from build123d import *

# Parameters (mm, degrees)
F0_W      = 50.8
F0_H      = 30.48
F1_DEPTH  = 25.4
F2_DEPTH  = 55.626
F3_DEPTH  = 32.766
F6_DEPTH  = 25.4
F7_DEPTH  = 25.4
F9_DEPTH  = 25.4
F10_DEPTH = 7.62


with BuildPart() as f1:
    # F0 (on Front) → F1 (new body)
    with BuildSketch(Plane.XZ):
        with Locations((-32.1067409651, 15.24)):
            Rectangle(F0_W, F0_H)
    extrude(amount=F1_DEPTH)

    # F2 (add): a face of the model
    f2_faces = [f1.faces().sort_by_distance(p)[0] for p in [
        (-32.1067409651, 0, 15.24),
    ]]
    extrude(f2_faces, amount=F2_DEPTH)

    # F3 (add): a face of the model
    f3_faces = [f1.faces().sort_by_distance(p)[0] for p in [
        (-6.7067409651, 15.113, 15.24),
    ]]
    extrude(f3_faces, amount=F3_DEPTH)

    # F4 (on face) → F6 (cut)
    with BuildSketch(Plane.XY.offset(30.48)):
        Polygon((-11.3192433491, -25.4), (17.2114539891, 55.626), (-57.5067409651, 55.626), (-57.5067409651, -25.4), align=None)
    extrude(amount=-F6_DEPTH, mode=Mode.SUBTRACT)

    # F5 (on face) → F7 (cut)
    with BuildSketch(Plane.XY.offset(30.48)):
        Polygon((-57.5067409651, -25.4), (-11.3192433491, -25.4), (17.2114539891, 55.626), (-43.2823600247, 55.626), (-57.5067409651, 55.626), align=None)
    extrude(amount=-F7_DEPTH, mode=Mode.SUBTRACT)

    # F8 (on face) → F9 (join)
    with BuildSketch(Plane.XY.offset(5.08)):
        Polygon((-57.5067409651, 20.3126166016), (-36.7487818003, 55.626), (-57.5067409651, 55.626), align=None)
    extrude(amount=F9_DEPTH)

    # F10 (add): a face of the model
    f10_faces = [f1.faces().sort_by_distance(p)[0] for p in [
        (-24.788870281, 16.2328343869, 5.08),
    ]]
    extrude(f10_faces, amount=F10_DEPTH)


solid = f1.part
Could you check a few things on this model? Use its own coordinates, in mm. A direction names the side the tool comes from. Give positions to 0.01 mm unless a question says otherwise; leave off trailing zeros. Order: outer loops, then holes, each group sorted by start corner. A loop starts at its lowest first (then second) coordinate and runs counter-clockwise, first axis right, second up. Notation, with made-up numbers: M -10.75,15 L 2.25,15 A14 cw 2.25,22 Z; hole C -32,61.5 d10. An arc over 180 degrees is marked long. One line per question, with ' | ' between items.
1. I want a section at C-C (x = -7). List the corners of the cut face in (y, z) for me.
Results:
outline: M -25.4,0 L 55.63,0 L 55.63,12.7 L -13.13,12.7 L -13.13,30.48 L -25.4,30.48 Z
2. I want a section at B-B (y = 34.5). List the corners of the cut face in (x, z) for me, and give its area (3 significant figures).
Results:
outline: M -57.51,0 L 26.06,0 L 26.06,30.48 L 9.77,30.48 L 9.77,12.7 L -49.17,12.7 L -49.17,30.48 L -57.51,30.48 Z | area: 1,500 mm²
3. If I drill on line 1 (X direction, y = 21, z = 17.5); line 2 (Z direction, x = -34.5, y = 7); line 3 (X direction, y = 48, z = 29), over which ranges is the centre line in solid material (lowest first)?
Results:
line 1: -57.51 to -57.1, 5.02 to 26.06 | line 2: 0 to 12.7 | line 3: -57.51 to -41.23, 14.53 to 26.06
4. I want a section at A-A (z = 16). List the corners of the cut face in (x, y) for me, and give its area (3 significant figures).
Results:
outline: M -57.51,20.31 L -36.75,55.63 L -57.51,55.63 Z; M -11.32,-25.4 L 26.06,-25.4 L 26.06,55.63 L 17.21,55.63 Z | area: 2,240 mm²
5. For faces 1 (the face through (-47.273, 37.722, 21.466)), 2 (the face through (2.746, 14.546, 21.714)), 3 (the face through (-15, 55.626, 12)), 4 (the face through (-21, 16, 12.7)), which set-ups out of +Z, -Z, +X, -X, +Y, -Y let a thin tool reach every point of the face, with its end or its side?
Results:
face 1: +Z, -Y | face 2: +Z, +Y | face 3: +Z, -Z, +X, -X, +Y | face 4: +Z
6. I want a section at D-D (y = 48). List the corners of the cut face in (x, z) for me.
Results:
outline: M -57.51,0 L 26.06,0 L 26.06,30.48 L 14.53,30.48 L 14.53,12.7 L -41.23,12.7 L -41.23,30.48 L -57.51,30.48 Z
7. I'm going to push a flat-ended pin straight in: pin 1 (1.5 mm diameter, centred on y = 12, z = 27.5, fed in from -X). Where does the tip first touch, or does it pass through?
Results:
pin 1: x = 1.59
